Could you check a few things on this model? Use its own coordinates, in mm. A direction names the side the tool comes from. Give positions to 0.01 mm unless a question says otherwise; leave off trailing zeros. Loops run counter-clockwise (first coordinate to the right, second up) from the corner with the lowest first, then second, coordinate; pieces in that order, holes last.
1. Imagine slicing it at C-C (z = 4.5). List the corners of the cut face in (x, y) for me, plus the area to 3 significant figures.
2. Imagine slicing it at D-D (y = 2.5). Count the separate pieces of the cut face and the enclosed holes in it, plus the area to 3 significant figures.
3. For P1, Ø2, axis at x = -15, z = 4.5, coming from the -Y side; P2, Ø4, axis at x = -3.5, z = 18, coming from the -Y side; P3, Ø10, axis at x = -12, z = -15.5, coming from the -Y side, each with a flat end and sliding along its axis, tell me the tip position at first contact or that it passes through.
4. I need wall thicknesses on line 1 along Z through (x, y) = (-8.25, 0.75); line 2 along Z through (x, y) = (-3.5, 3.25); line 3 along X through (y, z) = (3.75, 17.5). Which ranges of each line are inside material? Lowest first, please.
5. Imagine slicing it at B-B (z = 17.5). List the corners of the cut face in (x, y) for me, plus the area to 3 significant figures.
6. Thinking about a two-plate mould opening in Z: for faces 5 (the cylindrical face through (-9.9, 2.4, 14.8)), 6 (the flat face through (-10, 4.871, 0)), 7 (the flat face through (-5, 0, -12.25)), which applies, +Z half, -Z half, draft (parallel to the pull), parting line (faces both ways), or undercut?
7. For faces 1 (the flat face through (-13, 0, -19)), 2 (the cylindrical face through (-4.525, 2.522, 18.536)), 3 (the flat face through (-13, -0.12, 19)), 4 (the flat face through (-10.97, 2.41, 20.35)), which set-ups out of +Z, -Z, +X, -X, +Y, -Y let a thin tool reach every point of the face, with its end or its side?
8. Imagine slicing it at A-A (z = -17.5). List the corners of the cut face in (x, y) for me, plus the area to 3 significant figures.
```python
from build123d import *

# Parameters (mm, degrees)
BOSS_EXTRUDE1_DEPTH = 12.75
BOSS_EXTRUDE2_DEPTH = 24.5
BOSS_EXTRUDE3_DEPTH = 12.75
CUT_EXTRUDE1_DEPTH  = 34.504705063
CUT_EXTRUDE2_DEPTH  = 34.504705063


with BuildPart() as part:
    # Sketch1 → Boss-Extrude1 (new body)
    with BuildSketch(Plane(origin=(0, 0, -25), x_dir=(-1, 0, 0), z_dir=(0, 0, -1))):
        with BuildLine():
            Line((5.2, 0), (20.038095252, 0))
            Line((20.038095252, 0), (20.038095252, 4.871341922))
            Line((20.038095252, 4.871341922), (2.890551941, 4.871341922))
            ThreePointArc((2.890551941, 4.871341922), (2.649795512, 4.689964666), (2.757716863, 4.408514229))
            ThreePointArc((2.757716863, 4.408514229), (4.548633184, 2.519907966), (5.2, 0))
        make_face()
    extrude(amount=-BOSS_EXTRUDE1_DEPTH)

    # Sketch2 → Boss-Extrude2 (add)
    with BuildSketch(Plane.XY.offset(-12.25)):
        with BuildLine():
            Line((-20.038095252, 4.871341922), (-0.08660254, 4.871341922))
            ThreePointArc((-0.08660254, 4.871341922), (4.156921938, -2.478658078), (-4.330127019, -2.478658078))
            Line((-4.330127019, -2.478658078), (-20.038095252, 0.021341922))
            Line((-20.038095252, 0.021341922), (-20.038095252, 4.871341922))
        make_face()
    extrude(amount=BOSS_EXTRUDE2_DEPTH)

    # Sketch3 → Boss-Extrude3 (add)
    with BuildSketch(Plane.XY.offset(12.25)):
        with BuildLine():
            Line((-20.038095252, 4.871341922), (-2.767593084, 4.871341922))
            ThreePointArc((-2.767593084, 4.871341922), (-2.52626626, 4.686621046), (-2.641564255, 4.405432834))
            ThreePointArc((-2.641564255, 4.405432834), (-4.544193916, 2.489173945), (-5.24, -0.12002165))
            Line((-5.24, -0.12002165), (-20.038095252, -0.12002165))
            Line((-20.038095252, -0.12002165), (-20.038095252, 4.871341922))
        make_face()
    extrude(amount=BOSS_EXTRUDE3_DEPTH)

    # Sketch4 → Cut-Extrude1 (cut, through all)
    with BuildSketch(Plane(origin=(0, 4.871341922, 0), x_dir=(-1, 0, 0), z_dir=(0, 1, 0))):
        with BuildLine():
            Line((10, -13.681623382), (8.090811691, -15.590811691))
            ThreePointArc((8.090811691, -15.590811691), (10, -20.2), (11.909188309, -15.590811691))
            Line((11.909188309, -15.590811691), (10, -13.681623382))
        make_face()
    extrude(amount=-CUT_EXTRUDE1_DEPTH, mode=Mode.SUBTRACT)

    # Sketch5 → Cut-Extrude2 (cut, through all)
    with BuildSketch(Plane(origin=(0, 4.871341922, 0), x_dir=(-1, 0, 0), z_dir=(0, 1, 0))):
        with BuildLine():
            Line((10, 21.318376618), (8.090811691, 19.409188309))
            ThreePointArc((8.090811691, 19.409188309), (10, 14.8), (11.909188309, 19.409188309))
            Line((11.909188309, 19.409188309), (10, 21.318376618))
        make_face()
    extrude(amount=-CUT_EXTRUDE2_DEPTH, mode=Mode.SUBTRACT)

    # Sketch6 → Cut-Revolve1 (revolve, cut)
    with BuildSketch(Plane.XZ, mode=Mode.PRIVATE) as cut_revolve1_sk:
        with BuildLine():
            Line((4.1, 12.25), (0, 12.25))
            Line((0, 12.25), (0, -12.25))
            Line((0, -12.25), (4.182916362, -12.25))
            ThreePointArc((4.182916362, -12.25), (2.257265667, -0.006376751), (4.1, 12.25))
        make_face()
    revolve(cut_revolve1_sk.sketch.rotate(Axis((0, 0, 12.25), (0, 0, -1)), 180), axis=Axis((0, 0, 12.25), (0, 0, -1)), mode=Mode.SUBTRACT)


solid = part.part
```
Derived:
1. outline: (-20.04, 0.02) - (-4.33, -2.48) arc R4.9 ccw (long way) to (-0.09, 4.87) - (-20.04, 4.87) - close; hole circle Ø4.98 at (0, 0)
1. area: 153 mm2
2. separate pieces: 1
2. enclosed holes: 2
2. area: 880 mm2
3. P1: stops at y = -0.94
3. P2: stops at y = -0.12
3. P3: stops at y = -1.86
4. line 1: z = -25 to -19.56, -15.43 to 15.44, 19.57 to 25
4. line 2: z = -12.25 to 12.25
4. line 3: x = -20.04 to -12.7, -7.3 to -3.53
5. outline: (-20.04, -0.12) - (-12.7, -0.12) - (-12.7, 4.87) - (-20.04, 4.87) - close; (-7.3, -0.12) - (-5.24, -0.12) arc R5.24 cw to (-2.64, 4.41) arc R0.25 ccw to (-2.77, 4.87) - (-7.3, 4.87) - close
5. area: 51.6 mm2
6. face 5: undercut
6. face 6: draft
6. face 7: -Z half
7. face 1: -Z, +X, -X, -Y
7. face 2: +Z, +X, -Y
7. face 3: +Z, +X, -X, -Y
7. face 4: +Y, -Y
8. outline: (-20.04, 0) - (-12.7, 0) - (-12.7, 4.87) - (-20.04, 4.87) - close; (-7.3, 0) - (-5.2, 0) arc R5.2 cw to (-2.76, 4.41) arc R0.25 ccw to (-2.89, 4.87) - (-7.3, 4.87) - close
8. area: 50.3 mm2
